Part model, mm, in its own coordinate system. Face numbers are marked on the shaded views. A direction names the side the tool comes from. Give positions to 0.01 mm unless a question says otherwise; leave off trailing zeros. Loops run counter-clockwise (first coordinate to the right, second up) from the corner with the lowest first, then second, coordinate; pieces in that order, holes last. Notation, with made-up numbers: M 46.25,63 L 81.25,63 A6 cw 81.25,69 Z; hole C 35,45.5 d8. An arc over 180 degrees is marked long. Put each result on its own line as item: value. Start each with the question number.
```python
from build123d import *
from OCP.BRepFilletAPI import BRepFilletAPI_MakeChamfer

# Parameters (mm, degrees)
BOSS_EXTRUDE1_DEPTH      = 6.35
BOSS_EXTRUDE1_DEPTH_BACK = 6.35
SKETCH2_R                = 1.984375
CUT_EXTRUDE1_DEPTH       = 35
CHAMFER1_SIZE            = 0.2
CHAMFER1_SIZE2           = 0.99759701
SKETCH3_W                = 12.7
SKETCH3_H                = 12.7
BOSS_EXTRUDE2_DEPTH      = 27
SKETCH4_R                = 1.984375
CUT_EXTRUDE2_DEPTH       = 55.743127936


with BuildPart() as part:
    # Sketch1 → Boss-Extrude1 (new, two sides: drawn at the far end of the back side and taken through both)
    with BuildSketch(Plane.XY.offset(-BOSS_EXTRUDE1_DEPTH_BACK)):
        Polygon((-23.4085, 6.35), (-21.7705, 10.85), (-20.4865, 10.85), (-18.8485, 6.35), (-17.1255, 6.35), (-15.4875, 10.85), (-14.2035, 10.85), (-12.5655, 6.35), (-10.8425, 6.35), (-9.2045, 10.85), (-7.9205, 10.85), (-6.2825, 6.35), (-4.5595, 6.35), (-2.9215, 10.85), (-1.6375, 10.85), (0.0005, 6.35), (1.7235, 6.35), (3.3615, 10.85), (4.6455, 10.85), (6.2835, 6.35), (8.0065, 6.35), (9.6445, 10.85), (10.9285, 10.85), (12.5665, 6.35), (14.2895, 6.35), (18.8495, 6.35), (20.5725, 6.35), (25.1325, 6.35), (25.1325, -6.35), (-25.1325, -6.35), (-25.1325, 6.35), align=None)
    extrude(amount=BOSS_EXTRUDE1_DEPTH + BOSS_EXTRUDE1_DEPTH_BACK)

    # Sketch2 → Cut-Extrude1 (cut)
    with BuildSketch(Plane.ZY.offset(25.1325)):
        with Locations((0, 2.35)):
            Circle(SKETCH2_R)
    extrude(amount=-CUT_EXTRUDE1_DEPTH, mode=Mode.SUBTRACT)

    # Chamfer1: one chamfer whose edges measure the first distance from different faces: ONE call of the kernel's chamfer builder (chamfer() names one face for all edges)
    chamfer1_edges_1 = [part.edges().sort_by_distance(p)[0] for p in [
        (-21.7705, 10.85, 0),
        (-20.4865, 10.85, 0),
    ]]
    chamfer1_side_1 = [part.faces().sort_by_distance(p)[0] for p in [
        (-21.1285, 10.85, 0),
    ]]
    chamfer1_edges_2 = [part.edges().sort_by_distance(p)[0] for p in [
        (-15.4875, 10.85, 0),
        (-14.2035, 10.85, 0),
    ]]
    chamfer1_side_2 = [part.faces().sort_by_distance(p)[0] for p in [
        (-14.8455, 10.85, 0),
    ]]
    chamfer1_edges_3 = [part.edges().sort_by_distance(p)[0] for p in [
        (-9.2045, 10.85, 0),
        (-7.9205, 10.85, 0),
    ]]
    chamfer1_side_3 = [part.faces().sort_by_distance(p)[0] for p in [
        (-8.5625, 10.85, 0),
    ]]
    chamfer1_edges_4 = [part.edges().sort_by_distance(p)[0] for p in [
        (-2.9215, 10.85, 0),
        (-1.6375, 10.85, 0),
    ]]
    chamfer1_side_4 = [part.faces().sort_by_distance(p)[0] for p in [
        (-2.2795, 10.85, 0),
    ]]
    chamfer1_edges_5 = [part.edges().sort_by_distance(p)[0] for p in [
        (3.3615, 10.85, 0),
        (4.6455, 10.85, 0),
    ]]
    chamfer1_side_5 = [part.faces().sort_by_distance(p)[0] for p in [
        (4.0035, 10.85, 0),
    ]]
    chamfer1_edges_6 = [part.edges().sort_by_distance(p)[0] for p in [
        (9.6445, 10.85, 0),
        (10.9285, 10.85, 0),
    ]]
    chamfer1_side_6 = [part.faces().sort_by_distance(p)[0] for p in [
        (10.2865, 10.85, 0),
    ]]
    chamfer1 = BRepFilletAPI_MakeChamfer(part.part.solid().wrapped)
    for e in chamfer1_edges_1:
        chamfer1.Add(CHAMFER1_SIZE, CHAMFER1_SIZE2, e.wrapped, chamfer1_side_1[0].wrapped)  # the first distance lies on this face
    for e in chamfer1_edges_2:
        chamfer1.Add(CHAMFER1_SIZE, CHAMFER1_SIZE2, e.wrapped, chamfer1_side_2[0].wrapped)  # the first distance lies on this face
    for e in chamfer1_edges_3:
        chamfer1.Add(CHAMFER1_SIZE, CHAMFER1_SIZE2, e.wrapped, chamfer1_side_3[0].wrapped)  # the first distance lies on this face
    for e in chamfer1_edges_4:
        chamfer1.Add(CHAMFER1_SIZE, CHAMFER1_SIZE2, e.wrapped, chamfer1_side_4[0].wrapped)  # the first distance lies on this face
    for e in chamfer1_edges_5:
        chamfer1.Add(CHAMFER1_SIZE, CHAMFER1_SIZE2, e.wrapped, chamfer1_side_5[0].wrapped)  # the first distance lies on this face
    for e in chamfer1_edges_6:
        chamfer1.Add(CHAMFER1_SIZE, CHAMFER1_SIZE2, e.wrapped, chamfer1_side_6[0].wrapped)  # the first distance lies on this face
    add(Compound.cast(chamfer1.Shape()), mode=Mode.REPLACE)

    # Sketch3 → Boss-Extrude2 (add)
    with BuildSketch(Plane(origin=(25.1325, 0, 0), x_dir=(0, 0, -1), z_dir=(1, 0, 0))):
        Rectangle(SKETCH3_W, SKETCH3_H)
    extrude(amount=BOSS_EXTRUDE2_DEPTH)

    # Sketch4 → Cut-Extrude2 (cut, through all)
    with BuildSketch(Plane.XY.offset(6.35)):
        with Locations((12.1325, -2.35)):
            Circle(SKETCH4_R)
    extrude(amount=-CUT_EXTRUDE2_DEPTH, mode=Mode.SUBTRACT)


solid = part.part
```
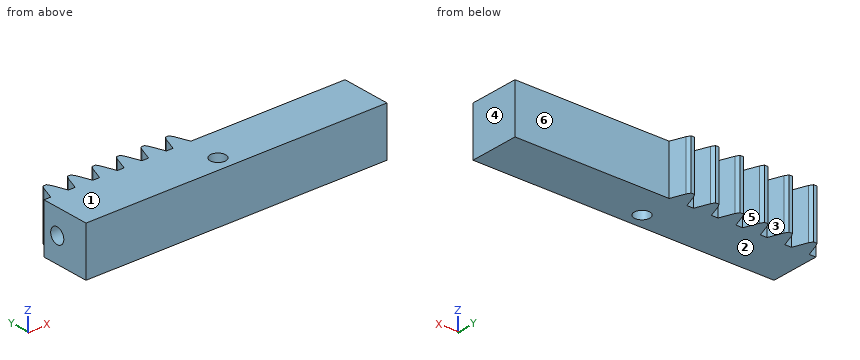
1) Band-saw the part on B-B on y = 8.75. Give the cut face in (x, z).
2) Pin check, flat tip, straight feed: pin 1 Ø6.5 at (x, z) = (25.5, 3) entering from +Y. Stop position of the tip, or through.
3) Band-saw the part on A-A on y = -2.35. Give the cut face in (x, z), then the cut area to 3 significant figures.
4) Wall check: L1, parallel to Y at x = -5.5, z = 0; L2, parallel to X at y = 9.75, z = 0.5; L3, parallel to X at y = 7.5, z = 6.25. Give the ranges that are in metal, low to high.
5) Band-saw the part on C-C on y = 2.35. Give the cut face in (x, z), then the cut area to 3 significant figures.
6) Which spindle directions (+Z, -Z, +X, -X, +Y, -Y) get a long thin tool onto all of the face, cutting with end or side? Do the marked faces 4, 5 and 6. Say none if no direction does.
7) Mould opens along Z. For the marked faces 1, 2 and 3 say: +Z half, -Z half, draft (parallel to the pull), parting line (faces both ways), or undercut.
8) Band-saw the part on D-D on x = 27.5. Give the cut face in (y, z).
Evaluation:
1. outline: M -22.53,-6.35 L -19.72,-6.35 L -19.72,6.35 L -22.53,6.35 Z; M -16.25,-6.35 L -13.44,-6.35 L -13.44,6.35 L -16.25,6.35 Z; M -9.97,-6.35 L -7.16,-6.35 L -7.16,6.35 L -9.97,6.35 Z; M -3.69,-6.35 L -0.87,-6.35 L -0.87,6.35 L -3.69,6.35 Z; M 2.6,-6.35 L 5.41,-6.35 L 5.41,6.35 L 2.6,6.35 Z; M 8.88,-6.35 L 11.69,-6.35 L 11.69,6.35 L 8.88,6.35 Z
2. pin 1: y = 6.35
3. outline: M -25.13,-6.35 L 10.15,-6.35 L 10.15,6.35 L -25.13,6.35 Z; M 14.12,-6.35 L 52.13,-6.35 L 52.13,6.35 L 14.12,6.35 Z
3. area: 931 mm2
4. L1: -6.35 to 0.37, 4.33 to 6.35
4. L2: -22.17 to -20.09, -15.89 to -13.8, -9.6 to -7.52, -3.32 to -1.24, 2.96 to 5.05, 9.24 to 11.33
4. L3: -22.99 to -19.27, -16.71 to -12.98, -10.42 to -6.7, -4.14 to -0.42, 2.14 to 5.86, 8.43 to 12.15
5. outline: M -25.13,-6.35 L 52.13,-6.35 L 52.13,6.35 L -25.13,6.35 L -25.13,1.98 L 9.87,1.98 L 9.87,-1.98 L -25.13,-1.98 Z
5. area: 842 mm2
6. face 4: +Z, -Z, +X, +Y, -Y
6. face 5: +Z, -Z, +Y
6. face 6: +Z, -Z, +X, +Y
7. face 1: +Z half
7. face 2: -Z half
7. face 3: draft
8. outline: M -6.35,-6.35 L 6.35,-6.35 L 6.35,6.35 L -6.35,6.35 Z
